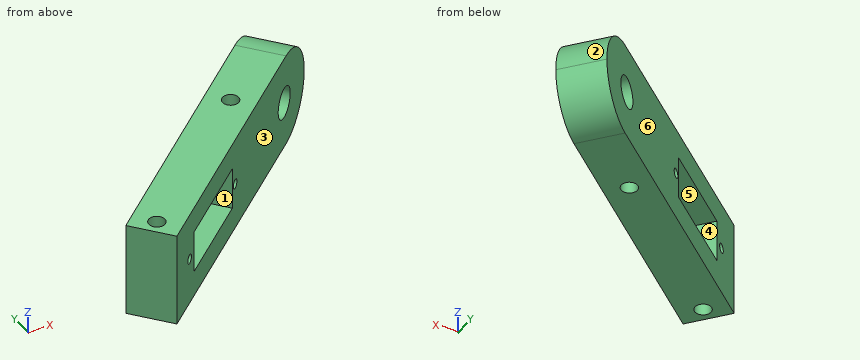
from build123d import *

# Parameters (mm, degrees)
SKETCH_1_W          = 70
SKETCH_1_H          = 20
SKETCH_1_W_2        = 21
SKETCH_1_H_2        = 9
EXTRUDE_1_DEPTH     = 10
CUT_EXTRUDE_1_REACH = 57.98
SKETCH_3_R          = 3.3
SKETCH_3_R_2        = 1
CUT_EXTRUDE_2_REACH = 60.746
SKETCH_4_R          = 1.7
FILLET_1_R          = 10


with BuildPart() as part:
    # 草图1 → 凸台-拉伸1 (new body)
    with BuildSketch(Plane(origin=(0, 0, 0), x_dir=(0.7660444431189771, 0.6427876096865406, 0), z_dir=(-0.6427876096865406, 0.7660444431189771, 0))):
        with Locations((15, 0)):
            Rectangle(SKETCH_1_W, SKETCH_1_H)
        Rectangle(SKETCH_1_W_2, SKETCH_1_H_2, mode=Mode.SUBTRACT)
    extrude(amount=EXTRUDE_1_DEPTH)

    # 草图3 → 切除-拉伸1 (cut, up to next)
    with BuildSketch(Plane(origin=(-6.427876097, 7.660444431, 0), x_dir=(0.7660444431189771, 0.6427876096865406, 0), z_dir=(-0.6427876096865405, 0.766044443118977, 0)), mode=Mode.PRIVATE) as cut_extrude_1_sk1:
        with Locations(Location((39, 0, 0), (0, 0, 180))):
            Circle(SKETCH_3_R)
    cut_extrude_1_tool1 = extrude(cut_extrude_1_sk1.sketch, amount=-CUT_EXTRUDE_1_REACH, mode=Mode.PRIVATE) & part.part
    # 草图3 → 切除-拉伸1 (cut, up to next)
    with BuildSketch(Plane(origin=(-6.427876097, 7.660444431, 0), x_dir=(0.7660444431189771, 0.6427876096865406, 0), z_dir=(-0.6427876096865405, 0.766044443118977, 0)), mode=Mode.PRIVATE) as cut_extrude_1_sk2:
        with Locations(Location((-13, 0, 0), (0, 0, 180))):
            Circle(SKETCH_3_R_2)
    cut_extrude_1_tool2 = extrude(cut_extrude_1_sk2.sketch, amount=-CUT_EXTRUDE_1_REACH, mode=Mode.PRIVATE) & part.part
    # 草图3 → 切除-拉伸1 (cut, up to next)
    with BuildSketch(Plane(origin=(-6.427876097, 7.660444431, 0), x_dir=(0.7660444431189771, 0.6427876096865406, 0), z_dir=(-0.6427876096865405, 0.766044443118977, 0)), mode=Mode.PRIVATE) as cut_extrude_1_sk3:
        with Locations(Location((12, 0, 0), (0, 0, 180))):
            Circle(SKETCH_3_R_2)
    cut_extrude_1_tool3 = extrude(cut_extrude_1_sk3.sketch, amount=-CUT_EXTRUDE_1_REACH, mode=Mode.PRIVATE) & part.part
    add(cut_extrude_1_tool1.solids().sort_by_distance((23.447857, 32.729161, 0))[0], mode=Mode.SUBTRACT)
    add(cut_extrude_1_tool2.solids().sort_by_distance((-16.386454, -0.695794, 0))[0], mode=Mode.SUBTRACT)
    add(cut_extrude_1_tool3.solids().sort_by_distance((2.764657, 15.373896, 0))[0], mode=Mode.SUBTRACT)

    # 草图4 → 切除-拉伸2 (cut, up to next)
    with BuildSketch(Plane.XY.offset(10), mode=Mode.PRIVATE) as cut_extrude_2_sk1:
        with Locations((-16.198218668, -7.064882864)):
            Circle(SKETCH_4_R)
    cut_extrude_2_tool1 = extrude(cut_extrude_2_sk1.sketch, amount=-CUT_EXTRUDE_2_REACH, mode=Mode.PRIVATE) & part.part
    # 草图4 → 切除-拉伸2 (cut, up to next)
    with BuildSketch(Plane.XY.offset(10), mode=Mode.PRIVATE) as cut_extrude_2_sk2:
        with Locations((14.862649296, 18.998279989)):
            Circle(SKETCH_4_R)
    cut_extrude_2_tool2 = extrude(cut_extrude_2_sk2.sketch, amount=-CUT_EXTRUDE_2_REACH, mode=Mode.PRIVATE) & part.part
    add(cut_extrude_2_tool1.solids().sort_by_distance((-16.198219, -7.064883, 10))[0], mode=Mode.SUBTRACT)
    add(cut_extrude_2_tool2.solids().sort_by_distance((14.862649, 18.99828, 10))[0], mode=Mode.SUBTRACT)

    # 圆角1
    fillet_1_edges = [part.edges().sort_by_distance(p)[0] for p in [
        (35.088284108, 35.9696027, -10),
        (35.088284108, 35.9696027, 10),
    ]]
    fillet(fillet_1_edges, radius=FILLET_1_R - 0.0001)  # a hair under: the kernel refuses the full size


solid = part.part
Check sheet for the modelled part. Datum: model origin and axes. Units: mm. Face numbers are marked on the shaded views. A direction names the side the tool comes from. Round coordinates to 2 decimals unless told otherwise and drop trailing zeros. Order: outer loops, then holes, each group sorted by start corner. A loop starts at its lowest first (then second) coordinate and runs counter-clockwise, first axis right, second up.
Q1. Cross-section at C-C, the plane x = -3.5. Enter the section's corners in (y, z).
Filled sheet:
outline: (-2.94, -10) - (10.12, -10) - (10.12, -4.5) - (-2.94, -4.5) - close; (-2.94, 4.5) - (10.12, 4.5) - (10.12, 10) - (-2.94, 10) - close
Q2. Set-up check for the marked faces 4, 5 and 6: record each of +Z, -Z, +X, -X, +Y, -Y from which the full face is reachable in a straight line by a thin tool's end or side.
Filled sheet:
face 4: +X, +Y
face 5: none
face 6: +Z, -Z, -X, +Y
Q3. Cross-section at A-A, the plane z = 2. Enter the section's corners in (x, y), plus the area to 3 significant figures.
Filled sheet:
outline: (-21.75, -5.2) - (-15.32, -12.86) - (-8.04, -6.75) - (-14.47, 0.91) - close; (1.62, 14.41) - (8.04, 6.75) - (27.86, 23.38) - (21.44, 31.04) - close; (25.46, 34.42) - (31.89, 26.76) - (38.15, 32.01) - (31.72, 39.67) - close; hole circle Ø3.4 at (-16.2, -7.06); hole circle Ø3.4 at (14.86, 19)
area: 417 mm2
Q4. Draft check along Z on the marked faces 1, 2 and 3. Enter one of: pulls with the +Z half, pulls with the -Z half, needs draft (parallel to the pull), parting line crosses it, or undercut.
Filled sheet:
face 1: undercut
face 2: pulls with the +Z half
face 3: needs draft
Q5. Cross-section at D-D, the plane z = 7. Enter the section's corners in (x, y).
Filled sheet:
outline: (-21.75, -5.2) - (-15.32, -12.86) - (36.11, 30.3) - (29.68, 37.96) - close; hole circle Ø3.4 at (-16.2, -7.06); hole circle Ø3.4 at (14.86, 19)
Q6. Cross-section at B-B, the plane y = 3.5. Enter the section's corners in (x, z).
Filled sheet:
outline: (-11.39, -10) - (4.17, -10) - (4.17, -4.5) - (-11.39, -4.5) - close; (-11.39, 4.5) - (4.17, 4.5) - (4.17, 10) - (-11.39, 10) - close
Q7. Depth check by flat-ended pin: P1, Ø1.5, axis at x = -11.5, z = -7.5, coming from the +Y side; P2, Ø3, axis at x = 11, z = -4, coming from the +Y side; P3, Ø8, axis at x = 3, y = -4.5, coming from the +Z side; P4, Ø8, axis at x = -8.5, z = 0, coming from the -Y side. Enter the tip coordinate at first touch or a pass-through.
Filled sheet:
P1: stops at y = 4.03
P2: stops at y = 23.54
P3: passes through
P4: stops at y = -10.49
Q8. Scan lines: L1, parallel to Z at x = -8.5, y = 5; L2, parallel to Z at x = 6, y = 10.5; L3, parallel to X at y = 20, z = 7.5. Record each from-to range of solid material in increasing order.
Filled sheet:
L1: z = -10 to -4.5, 4.5 to 10
L2: z = -10 to -0.76, 0.76 to 10
L3: x = 8.28 to 13.49, 16.24 to 23.84
